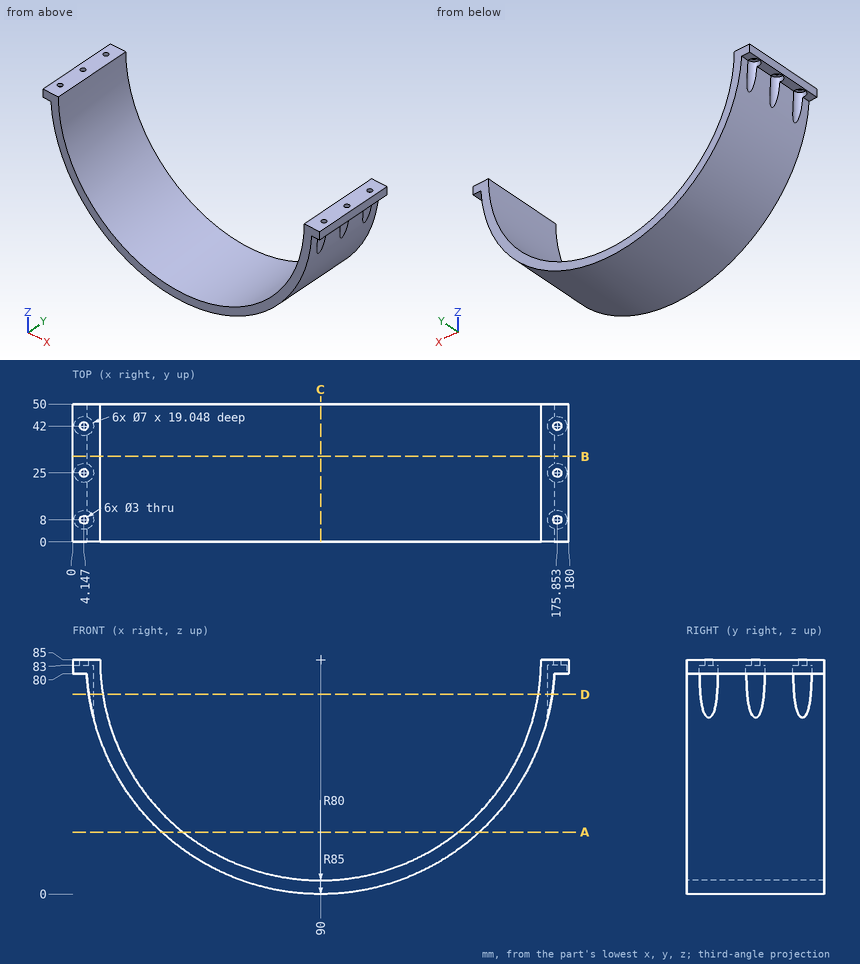
Print and shaded views of the part. All mm, measured from the part's lowest x, y and z. Give positions to 0.01 mm unless a question says otherwise; leave off trailing zeros. Order: outer loops, then holes, each group sorted by start corner. A loop starts at its lowest first (then second) coordinate and runs counter-clockwise, first axis right, second up. Notation, with made-up numbers: (18.25, 4) -> (32.25, 4) arc R19 ccw to (32.25, 39) -> close; hole circle Ø4 at (-31, -10.75). An arc over 180 degrees is marked (long way). Use CSV: the item, a comma, the result in double quotes.
1. Band-saw the part on C-C, the plane x = 90. Give the cut face in (y, z), then the cut area to 3 significant figures.
Outcome:
outline,"(0, 0) -> (50, 0) -> (50, 5) -> (0, 5) -> close"
area,"250 mm²"
2. Drop flat-ended pins along their axis: pin 1 (12 mm diameter, centred on y = 7, z = 63.5, fed in from +X); pin 2 (1.5 mm diameter, centred on x = 43.5, y = 25.5, fed in from -Z); pin 3 (3 mm diameter, centred on y = 28, z = 44.5, fed in from -X) (1 decimal). Give the stop position or say it passes through.
Outcome:
pin 1,"x = 173.53"
pin 2,"z = 13.36"
pin 3,"x = 14.5"
3. Band-saw the part on D-D, the plane z = 72.5. Give the cut face in (x, y) (1 decimal), then the cut area to 3 significant figures.
Outcome:
outline,"(5.9, 0) -> (11, 0) -> (11, 50) -> (5.9, 50) -> (5.9, 45) arc R3.5 cw to (5.9, 39) -> (5.9, 28) arc R3.5 cw to (5.9, 22) -> (5.9, 11) arc R3.5 cw to (5.9, 5) -> close; (169, 0) -> (174.1, 0) -> (174.1, 5) arc R3.5 cw to (174.1, 11) -> (174.1, 22) arc R3.5 cw to (174.1, 28) -> (174.1, 39) arc R3.5 cw to (174.1, 45) -> (174.1, 50) -> (169, 50) -> close"
area,"462 mm²"
4. Band-saw the part on A-A, the plane z = 22.5. Give the cut face in (x, y), then the cut area to 3 significant figures.
Outcome:
outline,"(32.39, 0) -> (40.06, 0) -> (40.06, 50) -> (32.39, 50) -> close; (139.94, 0) -> (147.61, 0) -> (147.61, 50) -> (139.94, 50) -> close"
area,"767 mm²"
5. Drill centre lines: line 1 along X through (y, z) = (22, 45.5) (1 decimal); line 2 along X through (y, z) = (35, 47.5); line 3 along Z through (x, y) = (123, 27). Where is each one in solid material? Low to high. Write a range as from..to.
Outcome:
line 1,"14.7..20.4, 159.6..165.3"
line 2,"13.72..19.33, 160.67..166.28"
line 3,"6.67..12.12"
6. Band-saw the part on B-B, the plane y = 31. Give the cut face in (x, z).
Outcome:
outline,"(0, 80) -> (5.15, 80) arc R85 ccw to (174.85, 80) -> (180, 80) -> (180, 85) -> (170, 85) arc R80 cw to (10, 85) -> (0, 85) -> close"
